```python
from build123d import *

# Parameters (mm, degrees)
AUFSATZ_LINEAR_AUSTRAGEN1_DEPTH = 2
AUFSATZ_LINEAR_AUSTRAGEN2_DEPTH = 22
SCHNITT_LINEAR_AUSTRAGEN1_REACH = 189.619
FASE1_SIZE                      = 1
FASE1_SIZE2                     = 3
SCHNITT_LINEAR_AUSTRAGEN2_REACH = 186.665
SKIZZE4_R                       = 1.7
SKIZZE5_R                       = 3.25
SCHNITT_LINEAR_AUSTRAGEN3_DEPTH = 3
SCHNITT_LINEAR_AUSTRAGEN4_REACH = 186.665


with BuildPart() as part:
    # Skizze1 → Aufsatz-Linear austragen1 (new body)
    with BuildSketch(Plane.XY):
        Polygon((-10, 10), (-95, 10), (-95, 160), (-105, 160), (-105, 0), (-10, 0), align=None)
    extrude(amount=AUFSATZ_LINEAR_AUSTRAGEN1_DEPTH)

    # Skizze2 → Aufsatz-Linear austragen2 (add)
    with BuildSketch(Plane.XY.offset(2)):
        Polygon((-105, 0), (-10, 0), (-10, 10), (-100, 10), (-100, 160), (-105, 160), align=None)
    extrude(amount=AUFSATZ_LINEAR_AUSTRAGEN2_DEPTH)

    # Skizze3 → Schnitt-Linear austragen1 (cut, up to next)
    with BuildSketch(Plane.ZY.offset(105), mode=Mode.PRIVATE) as schnitt_linear_austragen1_sk1:
        Polygon((3, 160), (24, 160), (24, 20), align=None)
    schnitt_linear_austragen1_tool1 = extrude(schnitt_linear_austragen1_sk1.sketch, amount=-SCHNITT_LINEAR_AUSTRAGEN1_REACH, mode=Mode.PRIVATE) & part.part
    add(schnitt_linear_austragen1_tool1.solids().sort_by_distance((-105, 113.333333, 17))[0], mode=Mode.SUBTRACT)

    # Fase1
    fase1_edges = [part.edges().sort_by_distance(p)[0] for p in [
        (-95, 85, 2),
    ]]
    fase1_side = [part.faces().sort_by_distance(p)[0] for p in [
        (-95, 85, 1),
    ]]
    chamfer(fase1_edges, length=FASE1_SIZE, length2=FASE1_SIZE2, reference=fase1_side[0])

    # Skizze4 → Schnitt-Linear austragen2 (cut, up to next)
    with BuildSketch(Plane(origin=(0, 10, 0), x_dir=(1, 0, 0), z_dir=(0, 1, 0)), mode=Mode.PRIVATE) as schnitt_linear_austragen2_sk1:
        with Locations(Location((-18, -19, 0), (0, 0, 270))):
            Circle(SKIZZE4_R)
    schnitt_linear_austragen2_tool1 = extrude(schnitt_linear_austragen2_sk1.sketch, amount=-SCHNITT_LINEAR_AUSTRAGEN2_REACH, mode=Mode.PRIVATE) & part.part
    # Skizze4 → Schnitt-Linear austragen2 (cut, up to next)
    with BuildSketch(Plane(origin=(0, 10, 0), x_dir=(1, 0, 0), z_dir=(0, 1, 0)), mode=Mode.PRIVATE) as schnitt_linear_austragen2_sk2:
        with Locations(Location((-27, -19, 0), (0, 0, 270))):
            Circle(SKIZZE4_R)
    schnitt_linear_austragen2_tool2 = extrude(schnitt_linear_austragen2_sk2.sketch, amount=-SCHNITT_LINEAR_AUSTRAGEN2_REACH, mode=Mode.PRIVATE) & part.part
    # Skizze4 → Schnitt-Linear austragen2 (cut, up to next)
    with BuildSketch(Plane(origin=(0, 10, 0), x_dir=(1, 0, 0), z_dir=(0, 1, 0)), mode=Mode.PRIVATE) as schnitt_linear_austragen2_sk3:
        with Locations(Location((-36, -19, 0), (0, 0, 270))):
            Circle(SKIZZE4_R)
    schnitt_linear_austragen2_tool3 = extrude(schnitt_linear_austragen2_sk3.sketch, amount=-SCHNITT_LINEAR_AUSTRAGEN2_REACH, mode=Mode.PRIVATE) & part.part
    add(schnitt_linear_austragen2_tool1.solids().sort_by_distance((-18, 10, 19))[0], mode=Mode.SUBTRACT)
    add(schnitt_linear_austragen2_tool2.solids().sort_by_distance((-27, 10, 19))[0], mode=Mode.SUBTRACT)
    add(schnitt_linear_austragen2_tool3.solids().sort_by_distance((-36, 10, 19))[0], mode=Mode.SUBTRACT)

    # Skizze5 → Schnitt-Linear austragen3 (cut)
    with BuildSketch(Plane(origin=(0, 10, 0), x_dir=(1, 0, 0), z_dir=(0, 1, 0))):
        with Locations(Location((-18, -19, 0), (0, 0, 180))):
            Circle(SKIZZE5_R)
        with Locations(Location((-27, -19, 0), (0, 0, 180))):
            Circle(SKIZZE5_R)
        with Locations(Location((-36, -19, 0), (0, 0, 180))):
            Circle(SKIZZE5_R)
    extrude(amount=-SCHNITT_LINEAR_AUSTRAGEN3_DEPTH, mode=Mode.SUBTRACT)

    # Skizze6 → Schnitt-Linear austragen4 (cut, up to next)
    with BuildSketch(Plane(origin=(0, 10, 0), x_dir=(1, 0, 0), z_dir=(0, 1, 0)), mode=Mode.PRIVATE) as schnitt_linear_austragen4_sk1:
        Polygon((-10, -10), (-10, 0), (-60, 0), (-45, -10), align=None)
    schnitt_linear_austragen4_tool1 = extrude(schnitt_linear_austragen4_sk1.sketch, amount=-SCHNITT_LINEAR_AUSTRAGEN4_REACH, mode=Mode.PRIVATE) & part.part
    # Skizze6 → Schnitt-Linear austragen4 (cut, up to next)
    with BuildSketch(Plane(origin=(0, 10, 0), x_dir=(1, 0, 0), z_dir=(0, 1, 0)), mode=Mode.PRIVATE) as schnitt_linear_austragen4_sk2:
        Polygon((-55, -24), (-70, -14), (-105, -14), (-105, -24), align=None)
    schnitt_linear_austragen4_tool2 = extrude(schnitt_linear_austragen4_sk2.sketch, amount=-SCHNITT_LINEAR_AUSTRAGEN4_REACH, mode=Mode.PRIVATE) & part.part
    add(schnitt_linear_austragen4_tool1.solids().sort_by_distance((-31.470588, 10, 4.705882))[0], mode=Mode.SUBTRACT)
    add(schnitt_linear_austragen4_tool2.solids().sort_by_distance((-83.529412, 10, 19.294118))[0], mode=Mode.SUBTRACT)


solid = part.part
```
Read the model definition and answer for the solid it produces. Units are mm, in the model's axes. A direction names the side the tool comes from. Give positions to 0.01 mm unless a question says otherwise; leave off trailing zeros. Loops run counter-clockwise (first coordinate to the right, second up) from the corner with the lowest first, then second, coordinate; pieces in that order, holes last.
Item 1: The mould has two halves that part along Z. Classify faces 1 (the flat face through (-62.395, 5.07, 19.07)), 2 (the cylindrical face through (-17.49, 3.55, 20.62)), 3 (the flat face through (-96, 63, 0)), 4 (the flat face through (-101, 160, 1)): released by +Z, released by -Z, zero draft, split by the parting line, or undercut.
Item 2: The part is cut by section C-C (z = 19). Give the number of separate pieces and of enclosed holes in the cut face, and give its area (3 significant figures).
Item 3: The part is cut by section B-B (y = 29). Write down the section's boundary in (x, z).
Item 4: The part is cut by section D-D (y = 73). Write down the section's boundary in (x, z).
Item 5: Each of these flat-tipped pins is pushed along its axis until it touches: pin 1 Ø2.5 at (x, z) = (-18, 19) entering from +Y; pin 2 Ø5 at (x, y) = (-95, 4.5) entering from +Z; pin 3 Ø5.5 at (x, z) = (-27, 19) entering from +Y; pin 4 Ø5 at (x, z) = (-19, 19) entering from +Y. Where does it stop, or does it pass through?
Item 6: For faces 5 (the flat face through (-28, 5, 10)), 6 (the flat face through (-102.535, 89.02, 13.647)), 7 (the flat face through (-19.4, 7, 17.6)), 8 (the flat face through (-100, 67, 10)), 9 (the flat face through (-103, 15, 24)), determine the directions among +Z, -Z, +X, -X, +Y, -Y from which every point of the face is accessible in a straight line to the end or side of a thin tool.
Item 7: Find the intervals of material crossed by line 1 along Z through (x, y) = (-18, 8.65); line 2 along X through (y, z) = (4, 19); line 3 along Y through (x, z) = (-95, 8.25), in increasing order.
Item 8: The part is cut by section A-A (x = -36). Write down the section's boundary in (y, z), and give its area (3 significant figures).
Taken from the geometry:
1. face 1: released by +Z
1. face 2: undercut
1. face 3: released by -Z
1. face 4: zero draft
2. separate pieces: 5
2. enclosed holes: 0
2. area: 612 mm2
3. outline: (-105, 0) - (-95, 0) - (-95, 1) - (-98, 2) - (-100, 2) - (-100, 22.65) - (-105, 22.65) - close
4. outline: (-105, 0) - (-95, 0) - (-95, 1) - (-98, 2) - (-100, 2) - (-100, 16.05) - (-105, 16.05) - close
5. pin 1: passes through
5. pin 2: stops at z = 14
5. pin 3: stops at y = 7
5. pin 4: stops at y = 10
6. face 5: -Z, +X, +Y, -Y
6. face 6: +Z, +X, -X, +Y
6. face 7: +Y
6. face 8: +Z, +X, +Y
6. face 9: +Z, +X, -X, +Y, -Y
7. line 1: z = 10 to 15.75, 22.25 to 24
7. line 2: x = -62.5 to -37.7, -34.3 to -28.7, -25.3 to -19.7, -16.3 to -10
7. line 3: y = 0 to 10
8. outline: (0, 10) - (10, 10) - (10, 15.75) - (7, 15.75) - (7, 17.3) - (0, 17.3) - close; (0, 20.7) - (7, 20.7) - (7, 22.25) - (10, 22.25) - (10, 24) - (0, 24) - close
8. area: 96.7 mm2
